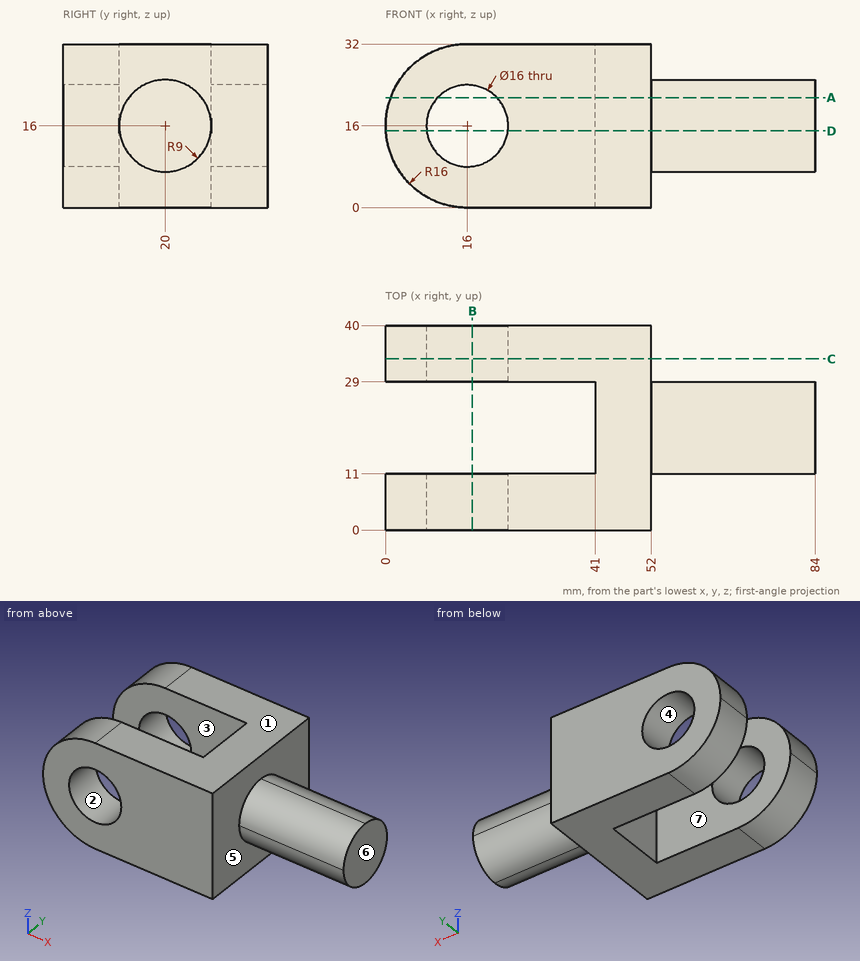
Drawing for the job (mm, zero at the part's lowest x, y, z). A direction names the side the tool comes from. Give positions to 0.01 mm unless a question says otherwise; leave off trailing zeros. Write each loop counter-clockwise with the first axis right and the second up, starting at its lowest first coordinate (ties: lowest second). Pieces come first, ordered by that corner, then holes. Notation, with made-up numbers: (-7, -38.75) -> (8, -38.75) arc R21 cw to (8, -15.75) -> close; hole circle Ø11 at (-26, -38.5). An arc over 180 degrees is marked (long way). Put each result on its own line as item: value. Start each with the question number.
Item 1: Pin check, flat tips, straight feed: pin 1 Ø6 at (x, y) = (37, 17.5) entering from +Z; pin 2 Ø5 at (y, z) = (11, 27.5) entering from +X; pin 3 Ø5 at (y, z) = (21.5, 7) entering from -X. Stop position of each tip, or through.
Item 2: Cut at B-B (x = 17). List the corners of the cut face in (y, z), then the cut area to 3 significant figures.
Item 3: Pull direction Z, two halves, no side cores. Call the marked faces 1, 2, 3 and 4: pulls with the +Z half, pulls with the -Z half, needs draft (parallel to the pull), parting line crosses it, or undercut.
Item 4: Cut at C-C (y = 33.5). List the corners of the cut face in (x, z).
Item 5: Wall check: L1, parallel to Z at x = 16, y = 3; L2, parallel to Y at x = 34.5, z = 21.5; L3, parallel to X at y = 17, z = 12. Give the ranges that are in metal, low to high. Write a range as [from, to].
Item 6: Cut at D-D (z = 15). List the corners of the cut face in (x, y).
Item 7: Cut at A-A (z = 21.5). List the corners of the cut face in (x, y), then the cut area to 3 significant figures.
Item 8: Which spindle directions (+Z, -Z, +X, -X, +Y, -Y) get a long thin tool onto all of the face, cutting with end or side? Do the marked faces 5, 6 and 7. Say none if no direction does.
Answer list:
1. pin 1: passes through
1. pin 2: stops at x = 52
1. pin 3: stops at x = 41
2. outline: (0, 0) -> (11, 0) -> (11, 8.06) -> (0, 8.06) -> close; (0, 23.94) -> (11, 23.94) -> (11, 32) -> (0, 32) -> close; (29, 0) -> (40, 0) -> (40, 8.06) -> (29, 8.06) -> close; (29, 23.94) -> (40, 23.94) -> (40, 32) -> (29, 32) -> close
2. area: 355 mm2
3. face 1: pulls with the +Z half
3. face 2: undercut
3. face 3: needs draft
3. face 4: undercut
4. outline: (16, 0) -> (52, 0) -> (52, 32) -> (16, 32) arc R16 ccw to start; hole circle Ø16 at (16, 16)
5. L1: z = [0, 8], [24, 32]
5. L2: y = [0, 11], [29, 40]
5. L3: x = [41, 84]
6. outline: (0.03, 0) -> (8.06, 0) -> (8.06, 11) -> (0.03, 11) -> close; (0.03, 29) -> (8.06, 29) -> (8.06, 40) -> (0.03, 40) -> close; (23.94, 0) -> (52, 0) -> (52, 11.06) -> (84, 11.06) -> (84, 28.94) -> (52, 28.94) -> (52, 40) -> (23.94, 40) -> (23.94, 29) -> (41, 29) -> (41, 11) -> (23.94, 11) -> close
7. outline: (0.98, 0) -> (10.19, 0) -> (10.19, 11) -> (0.98, 11) -> close; (0.98, 29) -> (10.19, 29) -> (10.19, 40) -> (0.98, 40) -> close; (21.81, 0) -> (52, 0) -> (52, 12.88) -> (84, 12.88) -> (84, 27.12) -> (52, 27.12) -> (52, 40) -> (21.81, 40) -> (21.81, 29) -> (41, 29) -> (41, 11) -> (21.81, 11) -> close
7. area: 1,520 mm2
8. face 5: +X
8. face 6: +Z, -Z, +X, +Y, -Y
8. face 7: +Z, -Z, -X
